```python
from build123d import *

# Parameters (mm, degrees)
SKETCH1_W           = 120
SKETCH1_H           = 100
BOSS_EXTRUDE1_DEPTH = 3.5
SKETCH9_R           = 3.825
CUT_EXTRUDE4_DEPTH  = 4
FILLET1_R           = 2
SKETCH10_R          = 3.75
BOSS_EXTRUDE4_DEPTH = 10
SKETCH11_R          = 7.5
BOSS_EXTRUDE5_DEPTH = 4
SKETCH12_R          = 7.5
BOSS_EXTRUDE6_DEPTH = 4
FILLET2_R           = 2
CUT_EXTRUDE9_DEPTH  = 2.5
FILLET3_R           = 1


with BuildPart() as part:
    # Sketch1 → Boss-Extrude1 (new body)
    with BuildSketch(Plane.XY):
        Rectangle(SKETCH1_W, SKETCH1_H)
    extrude(amount=BOSS_EXTRUDE1_DEPTH)

    # Sketch9 → Cut-Extrude4 (cut)
    with BuildSketch(Plane.XY.offset(3.5)):
        with Locations((46, 38)):
            Circle(SKETCH9_R)
    extrude(amount=-CUT_EXTRUDE4_DEPTH, mode=Mode.SUBTRACT)

    # Fillet1
    fillet1_edges = [part.edges().sort_by_distance(p)[0] for p in [
        (-60, 0, 3.5),
        (0, -50, 3.5),
        (60, 0, 3.5),
        (0, 50, 3.5),
    ]]
    fillet(fillet1_edges, radius=FILLET1_R)

    # Sketch10 → Boss-Extrude4 (add)
    with BuildSketch(Plane.XY.offset(3.5)):
        with Locations(Location((-40, -35, 0), (0, 0, 180))):
            Circle(SKETCH10_R)
        with Locations(Location((40, -35, 0), (0, 0, 180))):
            Circle(SKETCH10_R)
    extrude(amount=BOSS_EXTRUDE4_DEPTH)

    # Sketch11 → Boss-Extrude5 (add)
    with BuildSketch(Plane.XY.offset(13.5)):
        with Locations((-40, -35)):
            Circle(SKETCH11_R)
    extrude(amount=BOSS_EXTRUDE5_DEPTH)

    # Sketch12 → Boss-Extrude6 (add)
    with BuildSketch(Plane.XY.offset(13.5)):
        with Locations((40, -35)):
            Circle(SKETCH12_R)
    extrude(amount=BOSS_EXTRUDE6_DEPTH)

    # Fillet2
    fillet2_edges = [part.edges().sort_by_distance(p)[0] for p in [
        (-36.25, -35, 3.5),
        (43.75, -35, 3.5),
        (43.75, -35, 13.5),
        (-47.5, -35, 17.5),
        (32.5, -35, 17.5),
    ]]
    fillet(fillet2_edges, radius=FILLET2_R)

    # Sketch19 → Cut-Extrude9 (cut)
    with BuildSketch(Plane.XY.offset(3.5)):
        Polygon((-21.265387255, -30.401058823), (-25.887753182, -26.575652539), (-3.894109616, 1.04e-07), (-25.887751659, 26.575653799), (-21.265385732, 30.401060083), (1.26e-07, 4.705382708), (21.265387255, 30.401058823), (25.887753182, 26.575652539), (3.894109616, -1.04e-07), (25.887751659, -26.575653799), (21.265385732, -30.401060083), (-1.26e-07, -4.705382708), align=None)
    extrude(amount=-CUT_EXTRUDE9_DEPTH, mode=Mode.SUBTRACT)

    # Fillet3
    fillet3_edges = [part.edges().sort_by_distance(p)[0] for p in [
        (-3.894109616, 1.04e-07, 2.25),
        (-25.887751659, 26.575653799, 2.25),
        (-21.265385732, 30.401060083, 2.25),
        (1.26e-07, 4.705382708, 2.25),
        (21.265387255, 30.401058823, 2.25),
        (25.887753182, 26.575652539, 2.25),
        (3.894109616, -1.04e-07, 2.25),
        (25.887751659, -26.575653799, 2.25),
        (21.265385732, -30.401060083, 2.25),
        (-1.26e-07, -4.705382708, 2.25),
        (-21.265387255, -30.401058823, 2.25),
        (-25.887753182, -26.575652539, 2.25),
    ]]
    fillet(fillet3_edges, radius=FILLET3_R)


solid = part.part
```
The model under review builds one solid part; all positions refer to its coordinate system, in mm. A direction names the side the tool comes from. Round coordinates to 2 decimals unless told otherwise and drop trailing zeros. Loops run counter-clockwise (first coordinate to the right, second up) from the corner with the lowest first, then second, coordinate; pieces in that order, holes last. Notation, with made-up numbers: (-31, 3.25) -> (17, 3.25) arc R21 ccw to (17, 20.25) -> close; hole circle Ø7 at (12, 69.25). An arc over 180 degrees is marked (long way). Answer in a Markdown table with one row per item.
1) Tool access review of faces 3 (the flat face through (38, -41, 13.5)), 4 (the flat face through (10.56, 17.466, 2.268)), 5 (the flat face through (40, -35, 17.5)): name each direction out of +Z, -Z, +X, -X, +Y, -Y from which nothing blocks a thin tool from reaching the whole face with its end or side.
Taken from the geometry:
| item | result |
|---|---|
| face 3 | none |
| face 4 | +Z |
| face 5 | +Z, +X, -X, +Y, -Y |
2) For pin 1 Ø1.5 at (x, y) = (-19.5, 5) entering from -Z; pin 2 Ø1.5 at (x, y) = (-36.5, 4) entering from +Z; pin 3 Ø6 at (y, z) = (-16, 5) entering from +X, all flat-tipped, find the tip position at first contact; note any pin that passes through.
Taken from the geometry:
| item | result |
|---|---|
| pin 1 | stops at z = 0 |
| pin 2 | stops at z = 3.5 |
| pin 3 | stops at x = 59.94 |
3) Consider section A-A, the plane x = 40. Write out the cut boundary in (y, z), plus the area to 3 significant figures.
Taken from the geometry:
| item | result |
|---|---|
| outline | (-50, 0) -> (50, 0) -> (50, 1.5) arc R2 ccw to (48, 3.5) -> (-29.25, 3.5) arc R2 cw to (-31.25, 5.5) -> (-31.25, 11.5) arc R2 cw to (-29.25, 13.5) -> (-27.5, 13.5) -> (-27.5, 15.5) arc R2 ccw to (-29.5, 17.5) -> (-40.5, 17.5) arc R2 ccw to (-42.5, 15.5) -> (-42.5, 13.5) -> (-40.75, 13.5) arc R2 cw to (-38.75, 11.5) -> (-38.75, 5.5) arc R2 cw to (-40.75, 3.5) -> (-48, 3.5) arc R2 ccw to (-50, 1.5) -> close |
| area | 485 mm² |
4) Consider section C-C, the plane x = -49.5. Write out the cut boundary in (y, z), plus the area to 3 significant figures.
Taken from the geometry:
| item | result |
|---|---|
| outline | (-50, 0) -> (50, 0) -> (50, 1.5) arc R2 ccw to (48, 3.5) -> (-48, 3.5) arc R2 ccw to (-50, 1.5) -> close |
| area | 348 mm² |
5) Draft analysis for pull direction X (two halves, no side actions). For faces 1 (the cylindrical face through (38.27, -31.673, 8.458)), 2 (the flat face through (-1, 1, 0)), state which applies: pulls with the +X half, pulls with the -X half, needs draft (parallel to the pull), parting line crosses it, or undercut.
Taken from the geometry:
| item | result |
|---|---|
| face 1 | undercut |
| face 2 | needs draft |
6) Wall thickness on line 1 along Y through (x, z) = (46, 1.45) (3 decimals); line 2 along Z through (x, y) = (51, 20); line 3 along Z through (x, y) = (7.5, 4.5): over which ranges is each line inside the solid? List them lowest first.
Taken from the geometry:
| item | result |
|---|---|
| line 1 | y = -50 to 34.175, 41.825 to 50 |
| line 2 | z = 0 to 3.5 |
| line 3 | z = 0 to 1 |
7) Consider section D-D, the plane y = 11.5. Write out the cut boundary in (x, z).
Taken from the geometry:
| item | result |
|---|---|
| outline | (-60, 0) -> (60, 0) -> (60, 1.5) arc R2 ccw to (58, 3.5) -> (13.41, 3.5) -> (13.41, 1) -> (5.62, 1) -> (5.62, 3.5) -> (-5.62, 3.5) -> (-5.62, 1) -> (-13.41, 1) -> (-13.41, 3.5) -> (-58, 3.5) arc R2 ccw to (-60, 1.5) -> close |
